Drawing for the job (mm, zero at the part's lowest x, y, z). A direction names the side the tool comes from. Coordinates: 2 decimals unless noted, no trailing zeros. Loops run counter-clockwise (first coordinate to the right, second up) from the corner with the lowest first, then second, coordinate; pieces in that order, holes last. Notation, with made-up numbers: (64, -36) - (103, -36) arc R13 cw to (103, -23) - close; hole circle Ø3 at (-39.5, 72.25). An arc over 180 degrees is marked (long way). Put each result on its own line as item: value.
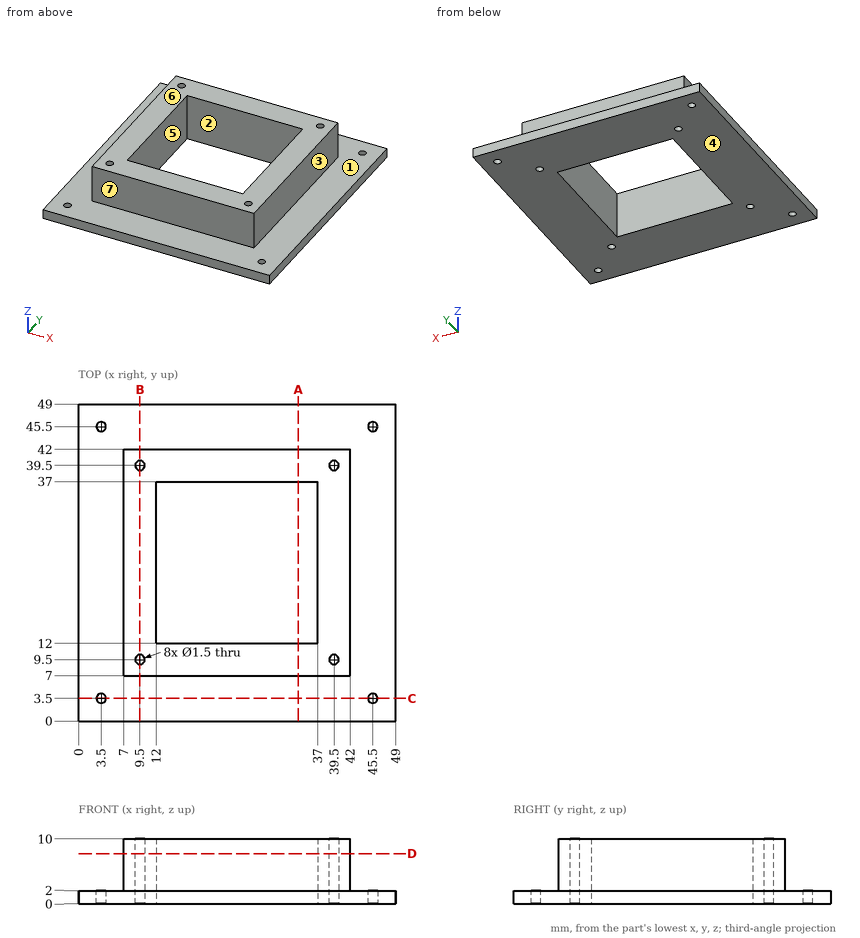
Q1. Wall check: L1, parallel to Y at x = 9.5, z = 5.75; L2, parallel to X at y = 45.5, z = 1.3. Give the ranges that are in metal, low to high. Write a range as from..to.
Determined:
L1: 7..8.75, 10.25..38.75, 40.25..42
L2: 0..2.75, 4.25..44.75, 46.25..49
Q2. Slice it at B-B, the plane x = 9.5. Give the cut face in (y, z).
Determined:
outline: (0, 0) - (8.75, 0) - (8.75, 10) - (7, 10) - (7, 2) - (0, 2) - close; (10.25, 0) - (38.75, 0) - (38.75, 10) - (10.25, 10) - close; (40.25, 0) - (49, 0) - (49, 2) - (42, 2) - (42, 10) - (40.25, 10) - close
Q3. Mould opens along Y. For the marked faces 5, 6 and 7 say: +Y half, -Y half, draft (parallel to the pull), parting line (faces both ways), or undercut.
Determined:
face 5: undercut
face 6: draft
face 7: -Y half
Q4. Slice it at C-C, the plane y = 3.5. Give the cut face in (x, z), then the cut area to 3 significant figures.
Determined:
outline: (0, 0) - (2.75, 0) - (2.75, 2) - (0, 2) - close; (4.25, 0) - (44.75, 0) - (44.75, 2) - (4.25, 2) - close; (46.25, 0) - (49, 0) - (49, 2) - (46.25, 2) - close
area: 92.0 mm2
Q5. Pin check, flat tips, straight feed: pin 1 Ø2.5 at (y, z) = (27, 4) entering from -X; pin 2 Ø1.2 at (x, y) = (39.5, 9.5) entering from +Z; pin 3 Ø2 at (x, y) = (3.5, 45.5) entering from +Z; pin 4 Ø3 at (y, z) = (30, 5.5) entering from +X. Stop position of each tip, or through.
Determined:
pin 1: x = 7
pin 2: through
pin 3: z = 2
pin 4: x = 42
Q6. Slice it at D-D, the plane z = 7.75. Give the cut face in (x, y).
Determined:
outline: (7, 7) - (42, 7) - (42, 42) - (7, 42) - close; hole circle Ø1.5 at (9.5, 9.5); hole circle Ø1.5 at (9.5, 39.5); hole (12, 12) - (37, 12) - (37, 37) - (12, 37) - close; hole circle Ø1.5 at (39.5, 9.5); hole circle Ø1.5 at (39.5, 39.5)
Q7. Slice it at A-A, the plane x = 34. Give the cut face in (y, z), then the cut area to 3 significant figures.
Determined:
outline: (0, 0) - (12, 0) - (12, 10) - (7, 10) - (7, 2) - (0, 2) - close; (37, 0) - (49, 0) - (49, 2) - (42, 2) - (42, 10) - (37, 10) - close
area: 128 mm2
Q8. Tool access for the marked faces 1, 2, 3 and 4: list every direction of +Z, -Z, +X, -X, +Y, -Y with a clear straight run to the whole face (end or side of a thin tool).
Determined:
face 1: +Z
face 2: +Z, -Z
face 3: +Z, +X, +Y, -Y
face 4: -Z, +X, -X, +Y, -Y
